```python
from build123d import *

# Parameters (mm, degrees)
SKETCH1_W            = 144
SKETCH1_H            = 134
SKETCH1_R            = 2
BOSS_EXTRUDE1_DEPTH  = 55
SKETCH2_R            = 2
CUT_EXTRUDE1_DEPTH   = 45
SKETCH3_W            = 144
SKETCH3_H            = 134
BOSS_EXTRUDE2_DEPTH  = 2
SKETCH5_R            = 2
BOSS_EXTRUDE4_DEPTH  = 4
SKETCH6_W            = 144
SKETCH6_H            = 134
SKETCH6_W_2          = 140
SKETCH6_H_2          = 130
BOSS_EXTRUDE5_DEPTH  = 10
BOSS_EXTRUDE11_DEPTH = 10
SKETCH12_R           = 1.5
CUT_EXTRUDE3_DEPTH   = 10


with BuildPart() as part:
    # Sketch1 → Boss-Extrude1 (new body)
    with BuildSketch(Plane(origin=(0, 0, 0), x_dir=(1, 0, 0), z_dir=(0, 1, 0))):
        Rectangle(SKETCH1_W, SKETCH1_H)
        with Locations((-62.5, 52.5)):
            Circle(SKETCH1_R, mode=Mode.SUBTRACT)
        with Locations((62.5, 52.5)):
            Circle(SKETCH1_R, mode=Mode.SUBTRACT)
        with Locations((-62.5, -52.5)):
            Circle(SKETCH1_R, mode=Mode.SUBTRACT)
        with Locations((62.5, -52.5)):
            Circle(SKETCH1_R, mode=Mode.SUBTRACT)
        with BuildLine():
            Line((-70, 65), (70, 65))
            Line((70, 65), (70, 57.5))
            Line((70, 57.5), (62.5, 57.5))
            ThreePointArc((62.5, 57.5), (57.5, 52.5), (62.5, 47.5))
            Line((62.5, 47.5), (70, 47.5))
            Line((70, 47.5), (70, -47.5))
            Line((70, -47.5), (62.5, -47.5))
            ThreePointArc((62.5, -47.5), (57.5, -52.5), (62.5, -57.5))
            Line((62.5, -57.5), (70, -57.5))
            Line((70, -57.5), (70, -65))
            Line((70, -65), (-70, -65))
            Line((-70, -65), (-70, -57.5))
            Line((-70, -57.5), (-62.5, -57.5))
            ThreePointArc((-62.5, -57.5), (-57.5, -52.5), (-62.5, -47.5))
            Line((-62.5, -47.5), (-70, -47.5))
            Line((-70, -47.5), (-70, 47.5))
            Line((-70, 47.5), (-62.5, 47.5))
            ThreePointArc((-62.5, 47.5), (-57.5, 52.5), (-62.5, 57.5))
            Line((-62.5, 57.5), (-70, 57.5))
            Line((-70, 57.5), (-70, 65))
        make_face(mode=Mode.SUBTRACT)
    extrude(amount=BOSS_EXTRUDE1_DEPTH)

    # Sketch2 → Cut-Extrude1 (cut)
    with BuildSketch(Plane(origin=(0, 55, 0), x_dir=(1, 0, 0), z_dir=(0, 1, 0))):
        with BuildLine():
            Line((-70, -47.5), (-62.5, -47.5))
            ThreePointArc((-62.5, -47.5), (-57.5, -52.5), (-62.5, -57.5))
            Line((-62.5, -57.5), (-70, -57.5))
            Line((-70, -57.5), (-70, -47.5))
        make_face()
        with Locations((-62.5, -52.5)):
            Circle(SKETCH2_R, mode=Mode.SUBTRACT)
        with BuildLine():
            Line((70, -57.5), (62.5, -57.5))
            ThreePointArc((62.5, -57.5), (57.5, -52.5), (62.5, -47.5))
            Line((62.5, -47.5), (70, -47.5))
            Line((70, -47.5), (70, -57.5))
        make_face()
        with Locations((62.5, -52.5)):
            Circle(SKETCH2_R, mode=Mode.SUBTRACT)
        with BuildLine():
            Line((70, 47.5), (62.5, 47.5))
            ThreePointArc((62.5, 47.5), (57.5, 52.5), (62.5, 57.5))
            Line((62.5, 57.5), (70, 57.5))
            Line((70, 57.5), (70, 47.5))
        make_face()
        with Locations((62.5, 52.5)):
            Circle(SKETCH2_R, mode=Mode.SUBTRACT)
        with BuildLine():
            Line((-62.5, 47.5), (-70, 47.5))
            Line((-70, 47.5), (-70, 57.5))
            Line((-70, 57.5), (-62.5, 57.5))
            ThreePointArc((-62.5, 57.5), (-57.5, 52.5), (-62.5, 47.5))
        make_face()
        with Locations((-62.5, 52.5)):
            Circle(SKETCH2_R, mode=Mode.SUBTRACT)
    extrude(amount=-CUT_EXTRUDE1_DEPTH, mode=Mode.SUBTRACT)

    # Sketch3 → Boss-Extrude2 (add)
    with BuildSketch(Plane.XZ):
        Rectangle(SKETCH3_W, SKETCH3_H)
    extrude(amount=BOSS_EXTRUDE2_DEPTH)

    # Sketch5 → Boss-Extrude4 (add)
    with BuildSketch(Plane.XZ.offset(2)):
        with BuildLine():
            Line((-70, -5), (-70, 5))
            Line((-70, 5), (-77, 5))
            ThreePointArc((-77, 5), (-82, 0), (-77, -5))
            Line((-77, -5), (-70, -5))
        make_face()
        with Locations((-77, 0)):
            Circle(SKETCH5_R, mode=Mode.SUBTRACT)
        with BuildLine():
            Line((5, -72), (5, -65))
            Line((5, -65), (-5, -65))
            Line((-5, -65), (-5, -72))
            ThreePointArc((-5, -72), (0, -77), (5, -72))
        make_face()
        with Locations((0, -72)):
            Circle(SKETCH5_R, mode=Mode.SUBTRACT)
        with BuildLine():
            Line((70, -5), (70, 5))
            Line((70, 5), (77, 5))
            ThreePointArc((77, 5), (82, 0), (77, -5))
            Line((77, -5), (70, -5))
        make_face()
        with Locations((77, 0)):
            Circle(SKETCH5_R, mode=Mode.SUBTRACT)
        with BuildLine():
            Line((-5, 65), (5, 65))
            Line((5, 65), (5, 72))
            ThreePointArc((5, 72), (0, 77), (-5, 72))
            Line((-5, 72), (-5, 65))
        make_face()
        with Locations((0, 72)):
            Circle(SKETCH5_R, mode=Mode.SUBTRACT)
    extrude(amount=-BOSS_EXTRUDE4_DEPTH)

    # Sketch6 → Boss-Extrude5 (add)
    with BuildSketch(Plane(origin=(0, 55, 0), x_dir=(1, 0, 0), z_dir=(0, 1, 0))):
        Rectangle(SKETCH6_W, SKETCH6_H)
        Rectangle(SKETCH6_W_2, SKETCH6_H_2, mode=Mode.SUBTRACT)
    extrude(amount=BOSS_EXTRUDE5_DEPTH)

    # Sketch11 → Boss-Extrude11 (add)
    with BuildSketch(Plane(origin=(0, 65, 0), x_dir=(1, 0, 0), z_dir=(0, 1, 0))):
        with BuildLine():
            ThreePointArc((-69, 67), (-74.121320344, 69.121320344), (-72, 64))
            Line((-72, 64), (-72, 65.5))
            ThreePointArc((-72, 65.5), (-73.060660172, 68.060660172), (-70.5, 67))
            Line((-70.5, 67), (-69, 67))
        make_face()
        with BuildLine():
            Line((72, 65.5), (72, 64))
            ThreePointArc((72, 64), (74.121320344, 69.121320344), (69, 67))
            Line((69, 67), (70.5, 67))
            ThreePointArc((70.5, 67), (72, 68.5), (73.5, 67))
            ThreePointArc((73.5, 67), (73.060660172, 65.939339828), (72, 65.5))
        make_face()
        with BuildLine():
            Line((70.5, -67), (69, -67))
            ThreePointArc((69, -67), (74.121320344, -69.121320344), (72, -64))
            Line((72, -64), (72, -65.5))
            ThreePointArc((72, -65.5), (73.060660172, -65.939339828), (73.5, -67))
            ThreePointArc((73.5, -67), (72, -68.5), (70.5, -67))
        make_face()
        with BuildLine():
            Line((-69, -67), (-70.5, -67))
            ThreePointArc((-70.5, -67), (-73.060660172, -68.060660172), (-72, -65.5))
            Line((-72, -65.5), (-72, -64))
            ThreePointArc((-72, -64), (-74.121320344, -69.121320344), (-69, -67))
        make_face()
    extrude(amount=-BOSS_EXTRUDE11_DEPTH)

    # Sketch12 → Cut-Extrude3 (cut)
    with BuildSketch(Plane(origin=(0, 65, 0), x_dir=(1, 0, 0), z_dir=(0, 1, 0))):
        with Locations((-72, 67)):
            Circle(SKETCH12_R)
        with Locations((72, 67)):
            Circle(SKETCH12_R)
        with Locations((72, -67)):
            Circle(SKETCH12_R)
        with Locations((-72, -67)):
            Circle(SKETCH12_R)
    extrude(amount=-CUT_EXTRUDE3_DEPTH, mode=Mode.SUBTRACT)


solid = part.part
```
Read the model definition and answer for the solid it produces. Units are mm, in the model's axes. A direction names the side the tool comes from. Give positions to 0.01 mm unless a question says otherwise; leave off trailing zeros. Order: outer loops, then holes, each group sorted by start corner. A loop starts at its lowest first (then second) coordinate and runs counter-clockwise, first axis right, second up.
(1) Find section B-B (x = 0). Give the vertices of the cut face in (y, z), plus the area to 3 significant figures.
(2) Find section A-A (y = 39). Give the vertices of the cut face in (x, z).
(3) Find section C-C (z = 0). Give the vertices of the cut face in (x, y), plus the area to 3 significant figures.
(4) Straight lines are drawn through the part: L1, parallel to Z at x = 44.5, y = 54.5; L2, parallel to X at y = 14, z = -49; L3, parallel to Z at x = 77, y = 0.3. For each, find the intervals that lie inside material, in ascending order.
(5) Given pin 1 (3 mm diameter, centred on x = -65, z = -53, fed in from +Y); pin 2 (4 mm diameter, centred on x = 54.5, y = 37, fed in from +Z); pin 3 (19.5 mm diameter, centred on y = 21.5, z = -26, fed in from -X), each flat-ended and moving along its own axis, determine where each tip first touches the part or whether it passes through.
(6) For a pull along X with two mould halves and no side action, classify faces 4 (the flat face through (-73.4, 55, -68.4)), 5 (the cylindrical face through (-75.092, -0.028, 0.601)), 6 (the cylindrical face through (82, 0, 0)) as released by +X, released by -X, zero draft, split by the parting line, or undercut.
(7) Find section D-D (x = -47.5). Give the vertices of the cut face in (y, z).
(8) For faces 1 (the flat face through (66, 5, -57.5)), 2 (the flat face through (5, 0, -70)), 3 (the flat face through (74, 0, 5)), determine the directions among +Z, -Z, +X, -X, +Y, -Y from which every point of the face is accessible in a straight line to the end or side of a thin tool.
Result sheet:
1. outline: (-2, -77) - (2, -77) - (2, -74) - (-2, -74) - close; (-2, -70) - (2, -70) - (2, -67) - (65, -67) - (65, -65) - (0, -65) - (0, 65) - (65, 65) - (65, 67) - (2, 67) - (2, 70) - (-2, 70) - close; (-2, 74) - (2, 74) - (2, 77) - (-2, 77) - close
1. area: 576 mm2
2. outline: (-72, -67) - (72, -67) - (72, 67) - (-72, 67) - close; hole (-70, -65) - (70, -65) - (70, 65) - (-70, 65) - close
3. outline: (-82, -2) - (-79, -2) - (-79, 2) - (-82, 2) - close; (-75, -2) - (75, -2) - (75, 2) - (72, 2) - (72, 65) - (70, 65) - (70, 0) - (-70, 0) - (-70, 65) - (-72, 65) - (-72, 2) - (-75, 2) - close; (79, -2) - (82, -2) - (82, 2) - (79, 2) - close
3. area: 596 mm2
4. L1: z = -67 to -65, 65 to 67
4. L2: x = -72 to -70, 70 to 72
4. L3: z = -5 to -2, 2 to 5
5. pin 1: stops at y = 10
5. pin 2: stops at z = 67
5. pin 3: stops at x = -72
6. face 4: zero draft
6. face 5: undercut
6. face 6: released by +X
7. outline: (-2, -67) - (65, -67) - (65, -65) - (0, -65) - (0, 65) - (65, 65) - (65, 67) - (-2, 67) - close
8. face 1: +Y
8. face 2: -Z, +X, +Y, -Y
8. face 3: +Z, +X, +Y, -Y
